```python
from build123d import *

# Parameters (mm, degrees)
F0_W     = 431.8
F0_H     = 355.6
F1_DEPTH = 6.35
F2_W     = 431.8
F2_H     = 63.5
F3_DEPTH = 254
F5_DEPTH = 431.801


with BuildPart() as f1:
    # F0 (on Front) → F1 (new body)
    with BuildSketch(Plane.XZ):
        with Locations((-215.9, 177.8)):
            Rectangle(F0_W, F0_H)
    extrude(amount=F1_DEPTH)

    # F2 (on Front) → F3 (join)
    with BuildSketch(Plane.XZ):
        with Locations((-215.9, -31.75)):
            Rectangle(F2_W, F2_H)
    extrude(amount=F3_DEPTH)

    # F4 (on Right) → F5 (cut, through all)
    with BuildSketch(Plane.YZ):
        Polygon((-330.205292, 41.198432), (-255.739987, -65.315232), (-172.791287, 61.935604), align=None)
    extrude(amount=-F5_DEPTH, mode=Mode.SUBTRACT)


solid = f1.part
```
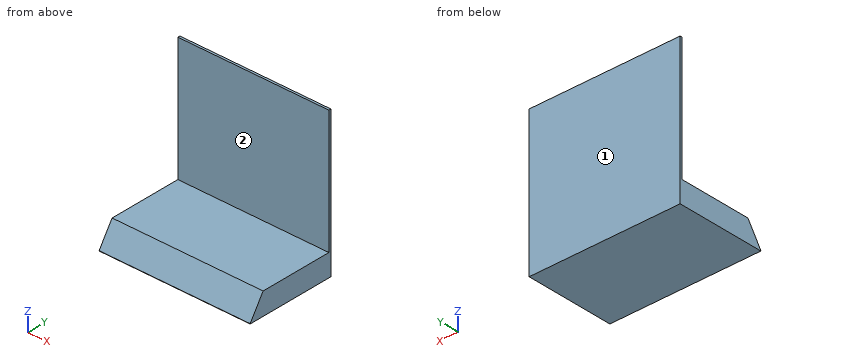
The model under review builds one solid part; all positions refer to its coordinate system, in mm. Face numbers are marked on the shaded views. A direction names the side the tool comes from. Round coordinates to 2 decimals unless told otherwise and drop trailing zeros. Loops run counter-clockwise (first coordinate to the right, second up) from the corner with the lowest first, then second, coordinate; pieces in that order, holes last. Notation, with made-up numbers: M -31,13 L 26,13 A11 ccw 26,23 Z; hole C 65,47.5 d9. An arc over 180 degrees is marked long. Answer as a JSON object with one key per item and string values.
(1) Take a section at B-B on z = 96. Give the boundary of the cut face in (x, y), and give its area (3 significant figures).
Resolved:
{"outline": "M -431.8,-6.35 L 0,-6.35 L 0,0 L -431.8,0 Z", "area": "2,740 mm²"}
(2) Tool access review of the marked faces 1 and 2: name each direction out of +Z, -Z, +X, -X, +Y, -Y from which nothing blocks a thin tool from reaching the whole face with its end or side.
Resolved:
{"face 1": "+Z, -Z, +X, -X, +Y", "face 2": "+Z, +X, -X, -Y"}
(3) Take a section at A-A on x = -396.5. Give the boundary of the cut face in (y, z).
Resolved:
{"outline": "M -254,-63.5 L 0,-63.5 L 0,355.6 L -6.35,355.6 L -6.35,0 L -213.16,0 L -254,-62.65 Z"}
(4) Clearance check with flat-ended pins moving along their axes: P1, Ø12, axis at x = -174.5, z = 81.5, coming from the -Y side; P2, Ø3, axis at x = -285, y = -73, coming from the +Z side. State where each tip first meets the part, or that it passes through.
Resolved:
{"P1": "y = -6.35", "P2": "z = 0"}
(5) Take a section at C-C on y = -107. Give the boundary of the cut face in (x, z).
Resolved:
{"outline": "M -431.8,-63.5 L 0,-63.5 L 0,0 L -431.8,0 Z"}
(6) To check wall thickness, follow line 1 along Z through (x, y) = (-150.5, -67); line 2 along Y through (x, z) = (-270.5, 19); line 3 along Z through (x, y) = (-412, -222.5). State the ranges of each line that lie inside material, in increasing order.
Resolved:
{"line 1": "-63.5 to 0", "line 2": "-6.35 to 0", "line 3": "-63.5 to -14.32"}
